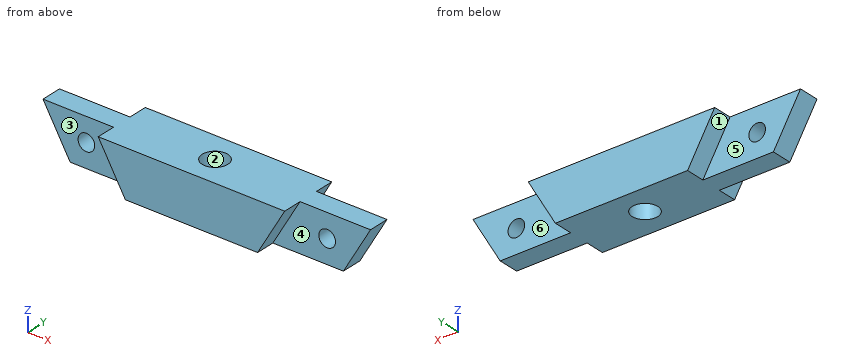
```python
from build123d import *

# Parameters (mm, degrees)
BOSS_EXTRUDE1_DEPTH = 7.9375
SKETCH5_R           = 3.4544
CUT_EXTRUDE2_DEPTH  = 30.30728297
SKETCH6_W           = 19.05
SKETCH6_H           = 5.55625
SKETCH7_W           = 19.05
SKETCH7_H           = 5.55625
CUT_EXTRUDE3_REACH  = 47.962
SKETCH8_R           = 2.2479


with BuildPart() as part:
    # Sketch2 → Boss-Extrude1 (new, symmetric)
    with BuildSketch(Plane(origin=(0, 0, 0), x_dir=(1, 0, 0), z_dir=(0, 1, 0))):
        Polygon((-17.859375, 6.35), (17.859375, 6.35), (25.191723419, -6.35), (-25.191723419, -6.35), align=None)
    extrude(amount=BOSS_EXTRUDE1_DEPTH, both=True)

    # Sketch5 → Cut-Extrude2 (cut, through all)
    with BuildSketch(Plane.XY.offset(6.35)):
        Circle(SKETCH5_R)
    extrude(amount=-CUT_EXTRUDE2_DEPTH, mode=Mode.SUBTRACT)

    # Sweep1: sweep along a curve in space
    with BuildLine() as sweep1_path:
        Line((-17.859375, 7.9375, -6.35), (-25.191723419, 7.9375, 6.35))
    # Sketch6 → Sweep1 (sweep)
    with BuildSketch(Plane.XY.offset(6.35)):
        with Locations((-34.716723419, 0)):
            Rectangle(SKETCH6_W, SKETCH6_H)
    sweep(path=sweep1_path.line)

    # Sweep2: sweep along a curve in space
    with BuildLine() as sweep2_path:
        Line((25.191723419, 7.9375, 6.35), (17.859375, 7.9375, -6.35))
    # Sketch7 → Sweep2 (sweep)
    with BuildSketch(Plane.XY.offset(6.35)):
        with Locations((34.716723419, 0)):
            Rectangle(SKETCH7_W, SKETCH7_H)
    sweep(path=sweep2_path.line)

    # Sketch8 → Cut-Extrude3 (cut, up to next)
    with BuildSketch(Plane(origin=(0, 2.778125, 0), x_dir=(1, 0, 0), z_dir=(0, 1, 0)), mode=Mode.PRIVATE) as cut_extrude3_sk1:
        with Locations(Location((-32.524071837, 0, 0), (0, 0, 180))):
            Circle(SKETCH8_R)
    cut_extrude3_tool1 = extrude(cut_extrude3_sk1.sketch, amount=-CUT_EXTRUDE3_REACH, mode=Mode.PRIVATE) & part.part
    # Sketch8 → Cut-Extrude3 (cut, up to next)
    with BuildSketch(Plane(origin=(0, 2.778125, 0), x_dir=(1, 0, 0), z_dir=(0, 1, 0)), mode=Mode.PRIVATE) as cut_extrude3_sk2:
        with Locations(Location((32.524071837, 0, 0), (0, 0, 180))):
            Circle(SKETCH8_R)
    cut_extrude3_tool2 = extrude(cut_extrude3_sk2.sketch, amount=-CUT_EXTRUDE3_REACH, mode=Mode.PRIVATE) & part.part
    add(cut_extrude3_tool1.solids().sort_by_distance((-32.524072, 2.778125, 0))[0], mode=Mode.SUBTRACT)
    add(cut_extrude3_tool2.solids().sort_by_distance((32.524072, 2.778125, 0))[0], mode=Mode.SUBTRACT)


solid = part.part
```
For this review, take the finished solid that the model builds, in its own axes (mm). Face numbers are marked on the shaded views. A direction names the side the tool comes from. Give positions to 0.01 mm unless a question says otherwise; leave off trailing zeros. Write each loop counter-clockwise with the first axis right and the second up, starting at its lowest first coordinate (ties: lowest second). Pieces come first, ordered by that corner, then holes. Notation, with made-up numbers: M 87.5,-31.75 L 102.5,-31.75 A15 ccw 102.5,-20.75 Z; hole C -26,55.5 d9. An arc over 180 degrees is marked long. One line per item, written item: value.
1) For line 1 (Z direction, x = -32.5, y = 1); line 2 (X direction, y = -1.5, z = 0.5); line 3 (Y direction, x = 0, z = 0.5), list the stretches that pass through material, from the lowest coordinate up. Write a range as from..to.
Results are:
line 1: z = -6.35..-2.25, 2.25..6.35
line 2: x = -40.86..-34.72, -30.33..-3.11, 3.11..30.33, 34.72..40.86
line 3: y = -7.94..-3.45, 3.45..7.94
2) Take a section at A-A, the plane z = 0. Write out the cut boundary in (x, y).
Results are:
outline: M -40.58,-2.78 L -34.77,-2.78 L -34.77,2.78 L -40.58,2.78 Z; M -30.28,-2.78 L -21.53,-2.78 L -21.53,-7.94 L 21.53,-7.94 L 21.53,-2.78 L 30.28,-2.78 L 30.28,2.78 L 21.53,2.78 L 21.53,7.94 L -21.53,7.94 L -21.53,2.78 L -30.28,2.78 Z; M 34.77,-2.78 L 40.58,-2.78 L 40.58,2.78 L 34.77,2.78 Z; hole C 0,0 d6.91
3) Take a section at D-D, the plane y = -4.5. Write out the cut boundary in (x, z), then the cut area to 3 significant figures.
Results are:
outline: M -25.19,6.35 L -17.86,-6.35 L 17.86,-6.35 L 25.19,6.35 Z
area: 547 mm²
4) Take a section at C-C, the plane z = -3.75. Write out the cut boundary in (x, y), then the cut area to 3 significant figures.
Results are:
outline: M -38.41,-2.78 L -19.36,-2.78 L -19.36,-7.94 L 19.36,-7.94 L 19.36,-2.78 L 38.41,-2.78 L 38.41,2.78 L 19.36,2.78 L 19.36,7.94 L -19.36,7.94 L -19.36,2.78 L -38.41,2.78 Z; hole C 0,0 d6.91
area: 789 mm²
5) For the marked faces 4, 5 and 6, list the 3-axis set-ups (+Z, -Z, +X, -X, +Y, -Y) from which the entire face can be reached by the end or side of a thin tool; tool diameter is ignored.
Results are:
face 4: -Z, +X, -Y
face 5: -Z, -X, +Y
face 6: -Z, +X, +Y
6) The part is to be moulded in two halves that separate along Y. For the marked faces 1, 2 and 3, say which applies: +Y half, -Y half, draft (parallel to the pull), parting line (faces both ways), or undercut.
Results are:
face 1: draft
face 2: undercut
face 3: -Y half
7) Take a section at B-B, the plane x = 0. Write out the cut boundary in (y, z), then the cut area to 3 significant figures.
Results are:
outline: M -7.94,-6.35 L -3.45,-6.35 L -3.45,6.35 L -7.94,6.35 Z; M 3.45,-6.35 L 7.94,-6.35 L 7.94,6.35 L 3.45,6.35 Z
area: 114 mm²
8) For P1, Ø1, axis at x = 24, y = -6, coming from the -Z side; P2, Ø4, axis at x = -32.5, z = -3, coming from the -Y side; P3, Ø1.5, axis at y = 1, z = 2.5, coming from the -X side, all flat-tipped, find the tip position at first contact; note any pin that passes through.
Results are:
P1: stops at z = 3.42
P2: stops at y = -2.78
P3: stops at x = -42.45
